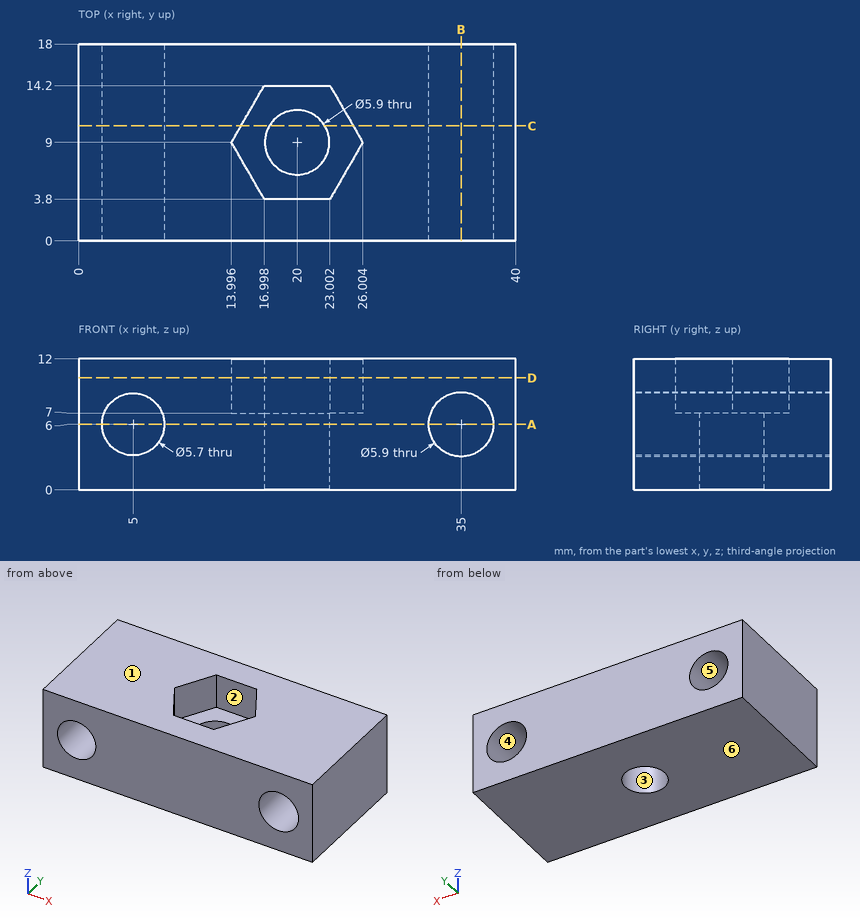
Source: three-view drawing plus pictorial views. Frame: mm from the lowest corner of the part. A direction names the side the tool comes from. Round coordinates to 2 decimals unless told otherwise and drop trailing zeros. Loops run counter-clockwise (first coordinate to the right, second up) from the corner with the lowest first, then second, coordinate; pieces in that order, holes last. Notation, with made-up numbers: M 21,-18.75 L 77,-18.75 A26 cw 77,-0.75 Z; hole C -40,89 d11. An arc over 180 degrees is marked long. Answer as CSV lines item,"result". Start each with the question number.
(1) Draft query along Z for the marked faces 3, 4, 5 and 6. Return one class per face: released by +Z, released by -Z, zero draft, split by the parting line, or undercut.
(2) Section D-D, the plane z = 10.25. Output: boundary loops of the cut face in (x, y) (1 decimal).
(3) Section A-A, the plane z = 6. Output: boundary loops of the cut face in (x, y), plus the area to 3 significant figures.
(4) Line query: line 1 (Z direction, x = 35, y = 13.75); line 2 (X direction, y = 7, z = 4.75); line 3 (Y direction, x = 20, z = 2.5). Output: solid intervals per line, ascending. Write a range as [from, to].
(5) Section B-B, the plane x = 35. Output: boundary loops of the cut face in (y, z), plus the area to 3 significant figures.
(6) Reachability of the marked faces 1 and 2 from +Z, -Z, +X, -X, +Y, -Y: full face, straight path, thin tool, end or side. Return the list, or none.
(7) Section C-C, the plane y = 10.5. Output: boundary loops of the cut face in (x, z), plus the area to 3 significant figures.
Values found:
1,face 3,"zero draft"
1,face 4,"undercut"
1,face 5,"undercut"
1,face 6,"released by -Z"
2,outline,"M 0,0 L 40,0 L 40,18 L 0,18 Z; hole M 14,9 L 17,3.8 L 23,3.8 L 26,9 L 23,14.2 L 17,14.2 Z"
3,outline,"M 0,0 L 2.15,0 L 2.15,18 L 0,18 Z; M 7.85,0 L 32.05,0 L 32.05,18 L 7.85,18 Z; M 37.95,0 L 40,0 L 40,18 L 37.95,18 Z; hole C 20,9 d5.9"
3,area,"484 mm²"
4,line 1,"z = [0, 3.05], [8.95, 12]"
4,line 2,"x = [0, 2.44], [7.56, 17.83], [22.17, 32.33], [37.67, 40]"
4,line 3,"y = [0, 6.05], [11.95, 18]"
5,outline,"M 0,0 L 18,0 L 18,3.05 L 0,3.05 Z; M 0,8.95 L 18,8.95 L 18,12 L 0,12 Z"
5,area,"110 mm²"
6,face 1,"+Z, +X, -X, +Y, -Y"
6,face 2,"+Z"
7,outline,"M 0,0 L 17.46,0 L 17.46,7 L 14.86,7 L 14.86,12 L 0,12 Z; M 22.54,0 L 40,0 L 40,12 L 25.14,12 L 25.14,7 L 22.54,7 Z; hole C 5,6 d5.7; hole C 35,6 d5.9"
7,area,"340 mm²"
